Here's the drawing with two shaded views (mm, measured from the low corner). I have some questions. Round coordinates to 2 decimals unless told otherwise and drop trailing zeros. Order: outer loops, then holes, each group sorted by start corner. A loop starts at its lowest first (then second) coordinate and runs counter-clockwise, first axis right, second up.
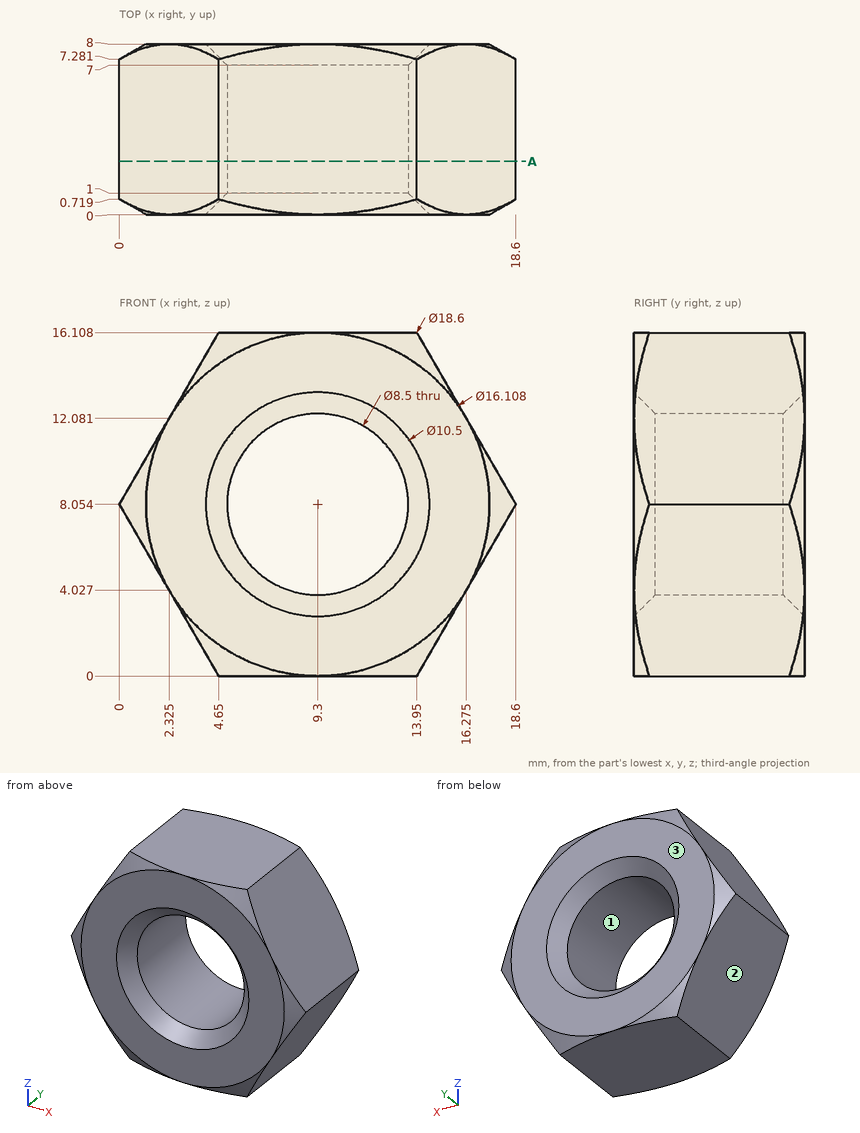
Q1. For P1, Ø3, axis at y = 6, z = 4.5, coming from the +X side (1 decimal); P2, Ø1, axis at y = 2, z = 5.5, coming from the -X side (1 decimal); P3, Ø2, axis at y = 5.5, z = 9, coming from the -X side; P4, Ø2, axis at x = 16.5, y = 2.5, coming from the +Z side (1 decimal), each with a flat end and sliding along its axis, tell me the tip position at first contact or that it passes through.
Q2. We'd pull the mould along X, two halves only. Please class the marked faces 1, 2 and 3: released by +X, released by -X, zero draft, split by the parting line, or undercut.
Q3. I need wall thicknesses on L1, parallel to Z at x = 9.5, y = 3; L2, parallel to Z at x = 10.25, y = 7.25 (1 decimal); L3, parallel to X at y = 2.75, z = 7. Which ranges of each line are inside material? Lowest first, please.
Q4. Imagine slicing it at A-A, the plane y = 2.5. Please give me the cut outline in (x, z).
Filled in:
1. P1: stops at x = 17.4
1. P2: stops at x = 1.2
1. P3: stops at x = 0
1. P4: stops at z = 13.4
2. face 1: undercut
2. face 2: released by -X
2. face 3: zero draft
3. L1: z = 0 to 3.81, 12.3 to 16.11
3. L2: z = 0 to 3.7, 12.5 to 16.1
3. L3: x = 0.61 to 5.18, 13.42 to 17.99
4. outline: (0, 8.05) - (4.65, 0) - (13.95, 0) - (18.6, 8.05) - (13.95, 16.11) - (4.65, 16.11) - close; hole circle Ø8.5 at (9.3, 8.05)
